Verification items for the finished model (mm, model axes). A direction names the side the tool comes from. Round coordinates to 2 decimals unless told otherwise and drop trailing zeros. Order: outer loops, then holes, each group sorted by start corner. A loop starts at its lowest first (then second) coordinate and runs counter-clockwise, first axis right, second up. Notation, with made-up numbers: M 28.5,-36 L 38.5,-36 A24 cw 38.5,-18 Z; hole C -2,25.5 d6. An arc over 180 degrees is marked long. One line per item, written item: value. Start each with the question number.
from build123d import *

# Parameters (mm, degrees)
M8_TAPPED_HOLE1_D     = 6.8
M8_TAPPED_HOLE1_DEPTH = 16
M8_TAPPED_HOLE1_TIP   = 2.042926105


with BuildPart() as part:
    # Sketch1 → Revolve1 (revolve)
    with BuildSketch(Plane.XY, mode=Mode.PRIVATE) as revolve1_sk:
        Polygon((-13, 0), (-13, 44), (-7, 44), (-7, 26), (0, 26), (0, 22), (-6.692307692, 22), (-6.692307692, 0), align=None)
    revolve(revolve1_sk.sketch.rotate(Axis((-37.153846154, 0, 0), (1, 0, 0)), 90), axis=Axis((-37.153846154, 0, 0), (1, 0, 0)))

    # M8 Tapped Hole1
    with Locations(Plane(origin=(-13, 0, -35), x_dir=(0, 0, -1), z_dir=(-1, 0, 0))):
        with Locations((0, 0), (-35, 35), (-70, 0), (-35, -35)):
            Hole(M8_TAPPED_HOLE1_D / 2, depth=M8_TAPPED_HOLE1_DEPTH)
            with Locations((0, 0, -(M8_TAPPED_HOLE1_DEPTH + M8_TAPPED_HOLE1_TIP / 2))):  # 118° drill point
                Cone(0, M8_TAPPED_HOLE1_D / 2, M8_TAPPED_HOLE1_TIP, mode=Mode.SUBTRACT)


solid = part.part
1. Section check C-C (y = 0). Record the cut outline in (x, z), and give its area (3 significant figures).
2. Draft check along Y on faces 3 (the face through (-7, 19, 19)), 4 (the face through (-9.96, 31.63, -0.44)), 5 (the face through (-3.451, 15.821, -20.633)). Enter one of: released by +Y, released by -Y, zero draft, split by the parting line, or undercut.
3. Scan lines: line 1 along Y through (x, z) = (-8.5, 0); line 2 along Y through (x, z) = (-10.3, -35); line 3 along Y through (x, z) = (-7.5, 32.5). Record each from-to range of solid material in increasing order.
4. Section check A-A (x = -9.25). Record the cut outline in (y, z).
5. Depth check by flat-ended pin: pin 1 (2 mm diameter, centred on x = -9.5, y = -20.5, fed in from +Z); pin 2 (6 mm diameter, centred on x = -11.5, y = 22.5, fed in from -Z); pin 3 (4 mm diameter, centred on y = 35, z = 0, fed in from +X); pin 4 (5 mm diameter, centred on x = -9.5, z = 14.5, fed in from +Y). Enter the tip coordinate at first touch or a pass-through.
6. Tool access check on faces 1 (the face through (-3.393, 21.477, -4.769)), 2 (the face through (-9.958, -1.021, -31.757)). Record the directions out of +Z, -Z, +X, -X, +Y, -Y that give a thin tool (end or side, any length) a straight path to the whole face; none if there is none.
7. Section check B-B (z = -35). Record the cut outline in (x, y).
Geometry check:
1. outline: M -13,-44 L -7,-44 L -7,-38.4 L -13,-38.4 Z; M -13,-31.6 L -7,-31.6 L -7,-26 L 0,-26 L 0,-22 L -6.69,-22 L -6.69,22 L 0,22 L 0,26 L -7,26 L -7,31.6 L -13,31.6 Z; M -13,38.4 L -7,38.4 L -7,44 L -13,44 Z
1. area: 516 mm²
2. face 3: zero draft
2. face 4: undercut
2. face 5: split by the parting line
3. line 1: y = -44 to -38.4, -31.6 to 31.6, 38.4 to 44
3. line 2: y = -26.66 to -3.4, 3.4 to 26.66
3. line 3: y = -29.66 to -2.3, 2.3 to 29.66
4. outline: C 0,0 d88; hole C -35,0 d6.8; hole C 0,-35 d6.8; hole C 0,35 d6.8; hole C 35,0 d6.8
5. pin 1: stops at z = 39.44
5. pin 2: stops at z = -39.44
5. pin 3: passes through
5. pin 4: stops at y = 42.33
6. face 1: +X
6. face 2: +X, -X
7. outline: M -13,-26.66 L -7,-26.66 L -7,-3.4 L -13,-3.4 Z; M -13,3.4 L -7,3.4 L -7,26.66 L -13,26.66 Z
